```python
from build123d import *

# Parameters (mm, degrees)
BOSS_EXTRUDE1_DEPTH = 15
CUT_EXTRUDE2_DEPTH  = 15
SKETCH4_W           = 15
SKETCH4_H           = 74
BOSS_EXTRUDE2_DEPTH = 10
SKETCH5_R           = 2.5
CUT_EXTRUDE3_DEPTH  = 10
SKETCH6_R           = 2.1
CUT_EXTRUDE4_DEPTH  = 16


with BuildPart() as part:
    # Sketch1 → Boss-Extrude1 (new body)
    with BuildSketch(Plane(origin=(0, 0, 0), x_dir=(0, 0, -1), z_dir=(1, 0, 0))):
        with BuildLine():
            Line((-37, 0), (-37, -200))
            Line((-37, -200), (37, -200))
            Line((37, -200), (37, 0))
            ThreePointArc((37, 0), (0, 37), (-37, 0))
        make_face()
    extrude(amount=BOSS_EXTRUDE1_DEPTH)

    # Sketch3 → Cut-Extrude2 (cut)
    with BuildSketch(Plane(origin=(15, 0, 0), x_dir=(0, 0, -1), z_dir=(1, 0, 0))):
        with BuildLine():
            Line((9.845321657, 9.230794756), (9.85, -29.35))
            ThreePointArc((9.85, -29.35), (9.672784276, -29.815555418), (9.230794756, -30.045321657))
            Line((9.230794756, -30.045321657), (-9.230794756, -30.045321657))
            ThreePointArc((-9.230794756, -30.045321657), (-9.665330895, -29.865330895), (-9.845321657, -29.430794756))
            Line((-9.845321657, -29.430794756), (-9.845321657, 9.230794756))
            ThreePointArc((-9.845321657, 9.230794756), (-9.665330895, 9.665330895), (-9.230794756, 9.845321657))
            Line((-9.230794756, 9.845321657), (9.230794756, 9.845321657))
            ThreePointArc((9.230794756, 9.845321657), (9.665330895, 9.665330895), (9.845321657, 9.230794756))
        make_face()
    extrude(amount=-CUT_EXTRUDE2_DEPTH, mode=Mode.SUBTRACT)

    # Sketch4 → Boss-Extrude2 (add)
    with BuildSketch(Plane.XZ.offset(200)):
        with Locations((-7.5, 0)):
            Rectangle(SKETCH4_W, SKETCH4_H)
    extrude(amount=-BOSS_EXTRUDE2_DEPTH)

    # Sketch5 → Cut-Extrude3 (cut)
    with BuildSketch(Plane(origin=(0, -190, 0), x_dir=(1, 0, 0), z_dir=(0, 1, 0))):
        with Locations((-7.5, 29.5)):
            Circle(SKETCH5_R)
        with Locations((-7.5, -29.5)):
            Circle(SKETCH5_R)
    extrude(amount=-CUT_EXTRUDE3_DEPTH, mode=Mode.SUBTRACT)

    # Sketch6 → Cut-Extrude4 (cut, through all)
    with BuildSketch(Plane.ZY):
        with Locations((4.925, 14.611145618)):
            Circle(SKETCH6_R)
        with Locations((-4.925, 14.611145618)):
            Circle(SKETCH6_R)
        with Locations((4.925, -34.811145618)):
            Circle(SKETCH6_R)
        with Locations((-4.925, -34.811145618)):
            Circle(SKETCH6_R)
    extrude(amount=-CUT_EXTRUDE4_DEPTH, mode=Mode.SUBTRACT)


solid = part.part
```
CAD build for the part. Positions are in the model's coordinates, mm. A direction names the side the tool comes from. Round coordinates to 2 decimals unless told otherwise and drop trailing zeros. Order: outer loops, then holes, each group sorted by start corner. A loop starts at its lowest first (then second) coordinate and runs counter-clockwise, first axis right, second up. Notation, with made-up numbers: (22, 82) -> (36, 82) arc R23 cw to (36, 106) -> close; hole circle Ø9 at (29.25, -5). An arc over 180 degrees is marked (long way). Write item = value, one per line.
(1) Cut at A-A (x = -7.5). Write the cut outline in (y, z).
Answers follow:
outline = (-200, -37) -> (-190, -37) -> (-190, -32) -> (-200, -32) -> close; (-200, -27) -> (-190, -27) -> (-190, 27) -> (-200, 27) -> close; (-200, 32) -> (-190, 32) -> (-190, 37) -> (-200, 37) -> close
(2) 3-axis set-ups, long thin cutter, end or side, ignore diameter. For faces 1 (the flat face through (0, -75, 1)), 2 (the flat face through (8, -10, 9.845)), 3 (the flat face through (6, -101, -37)): which of +Z, -Z, +X, -X, +Y, -Y reach the whole face in a straight line?
Answers follow:
face_1 = +Z, -Z, -X, +Y
face_2 = +X, -X
face_3 = -Z, +X, -X, +Y, -Y
(3) Cut at C-C (x = 10.25). Write the cut outline in (y, z) (3 decimals), plus the area to 3 significant figures.
Answers follow:
outline = (-200, -37) -> (0, -37) arc R37 ccw to (0, 37) -> (-200, 37) -> close; hole circle Ø4.2 at (-34.811, -4.925); hole circle Ø4.2 at (-34.811, 4.925); hole (-30.045, -9.231) arc R0.7 ccw to (-29.35, -9.85) -> (9.231, -9.845) arc R0.615 ccw to (9.845, -9.231) -> (9.845, 9.231) arc R0.615 ccw to (9.231, 9.845) -> (-29.431, 9.845) arc R0.615 ccw to (-30.045, 9.231) -> close; hole circle Ø4.2 at (14.611, -4.925); hole circle Ø4.2 at (14.611, 4.925)
area = 16,100 mm²
(4) Drill centre lines: L1, parallel to Z at x = -7.5, y = -197; L2, parallel to X at y = -192.5, z = -29.5; L3, parallel to Y at x = -4, z = -6. Where is each one in solid material? Low to high.
Answers follow:
L1 = -37 to -32, -27 to 27, 32 to 37
L2 = -15 to -10, -5 to 15
L3 = -200 to -190
(5) Pull direction Y, two halves, no side cores. Call faces 4 (the flat face through (15, -80, 1)), 5 (the cylindrical face through (7.4, 36.99, -0.81)), 6 (the cylindrical face through (7.395, 13.807, 6.865)), 7 (the flat face through (0, -200, 1)): +Y half, -Y half, draft (parallel to the pull), parting line (faces both ways), or undercut.
Answers follow:
face_4 = draft
face_5 = +Y half
face_6 = undercut
face_7 = -Y half
(6) Flat gauge pins, fed straight in: P1, Ø16.5, axis at x = -10, z = 18, coming from the +Y side; P2, Ø4.5, axis at x = 11, z = -4, coming from the +Y side; P3, Ø5.5, axis at y = -34.81, z = -4.92, coming from the -X side. Where does each tip first touch, or does it go through?
Answers follow:
P1 = -190
P2 = 36.96
P3 = 0
(7) Cut at B-B (z = -29.5). Write the cut outline in (x, y), plus the area to 4 significant figures.
Answers follow:
outline = (-15, -200) -> (-10, -200) -> (-10, -190) -> (-15, -190) -> close; (-5, -200) -> (15, -200) -> (15, 22.33) -> (0, 22.33) -> (0, -190) -> (-5, -190) -> close
area = 3,435 mm²
(8) Cut at D-D (y = -133). Write the cut outline in (x, z).
Answers follow:
outline = (0, -37) -> (15, -37) -> (15, 37) -> (0, 37) -> close
